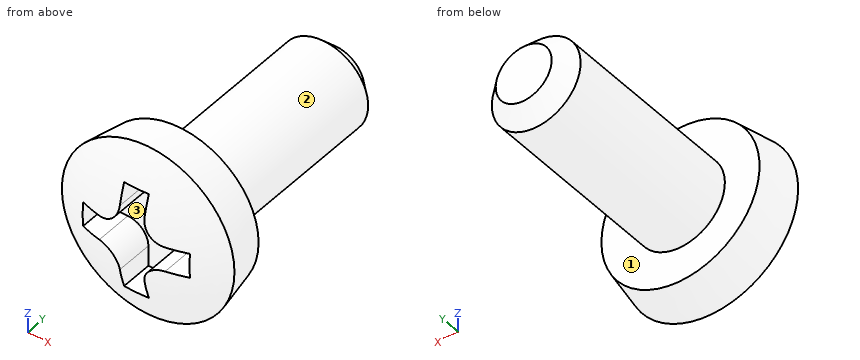
```python
from build123d import *

# Parameters (mm, degrees)
SKETCH1_R           = 2.667
BOSS_EXTRUDE1_DEPTH = 1.27
BOSS_EXTRUDE1_TAPER = 10
SKETCH3_R           = 1.3716
BOSS_EXTRUDE2_DEPTH = 6.35
CHAMFER1_SIZE       = 0.508
CUT_EXTRUDE5_DEPTH  = 3.048
FILLET1_R           = 0.635


with BuildPart() as part:
    # Sketch1 → Boss-Extrude1 (new body)
    with BuildSketch(Plane(origin=(0, 0, 0), x_dir=(1, 0, 0), z_dir=(0, 1, 0))):
        Circle(SKETCH1_R)
    extrude(amount=BOSS_EXTRUDE1_DEPTH, taper=BOSS_EXTRUDE1_TAPER)

    # Sketch2 → Revolve1 (revolve)
    with BuildSketch(Plane(origin=(0, 0, 0), x_dir=(0, 0, -1), z_dir=(1, 0, 0))):
        with BuildLine():
            Line((0, 0), (0, -0.762))
            ThreePointArc((0, -0.762), (-1.387624328, -0.57043515), (-2.667, 0))
            Line((-2.667, 0), (0, 0))
        make_face()
    revolve(axis=Axis((0, 0, 0), (0, -1, 0)))

    # Sketch3 → Boss-Extrude2 (add)
    with BuildSketch(Plane(origin=(0, 1.27, 0), x_dir=(1, 0, 0), z_dir=(0, 1, 0))):
        with Locations(Location((0, 0, 0), (0, 0, 270))):
            Circle(SKETCH3_R)
    extrude(amount=BOSS_EXTRUDE2_DEPTH)

    # Chamfer1
    chamfer1_edges = [part.edges().sort_by_distance(p)[0] for p in [
        (0, 7.62, -1.3716),
    ]]
    chamfer(chamfer1_edges, length=CHAMFER1_SIZE)

    # Sketch4 → Cut-Extrude5 (cut)
    with BuildSketch(Plane(origin=(0, -2.54, 0), x_dir=(1, 0, 0), z_dir=(0, 1, 0))):
        Polygon((-1.651, 0.381), (-1.651, -0.381), (-0.381, -0.381), (-0.381, -1.651), (0.381, -1.651), (0.381, -0.381), (1.651, -0.381), (1.651, 0.381), (0.381, 0.381), (0.381, 1.651), (-0.381, 1.651), (-0.381, 0.381), align=None)
    extrude(amount=CUT_EXTRUDE5_DEPTH, mode=Mode.SUBTRACT)

    # Fillet1
    fillet1_edges = [part.edges().sort_by_distance(p)[0] for p in [
        (0.381, -0.113446581, -0.381),
        (-0.381, -0.113446581, -0.381),
        (0.381, -0.113446581, 0.381),
        (-0.381, -0.113446581, 0.381),
    ]]
    fillet(fillet1_edges, radius=FILLET1_R)


solid = part.part
```
Read the model definition and answer for the solid it produces. Units are mm, in the model's axes. Face numbers are marked on the shaded views. Coordinates: 2 decimals unless noted, no trailing zeros. Loops run counter-clockwise (first coordinate to the right, second up) from the corner with the lowest first, then second, coordinate; pieces in that order, holes last. Notation, with made-up numbers: (17.5, 30.5) - (56.5, 30.5) arc R35 ccw to (56.5, 63.5) - close; hole circle Ø4 at (-11.5, 51.5). An arc over 180 degrees is marked (long way). Answer in a Markdown table with one row per item.
1. Straight lines are drawn through the part: line 1 (Z direction, x = -1.25, y = 0.25); line 2 (Y direction, x = -0.75, z = -0.05); line 3 (Y direction, x = 1.6, z = -0.7). For each, find the intervals that lie inside material, in ascending order.
Conclusion:
| item | result |
|---|---|
| line 1 | z = -2.31 to -0.38, 0.38 to 2.31 |
| line 2 | y = 0.51 to 7.62 |
| line 3 | y = -0.45 to 1.27 |
2. Find section A-A, the plane y = 1.75. Write down the section's boundary in (x, z).
Conclusion:
| item | result |
|---|---|
| outline | circle Ø2.74 at (0, 0) |
3. Determine the mould class of the marked faces 1, 2 and 3 for opening direction X: +X half, -X half, draft (parallel to the pull), parting line (faces both ways), or undercut.
Conclusion:
| item | result |
|---|---|
| face 1 | draft |
| face 2 | parting line |
| face 3 | undercut |
4. Given pin 1 (2 mm diameter, centred on x = 2, z = -1, fed in from -Y); pin 2 (1.5 mm diameter, centred on x = -1.5, y = 5, fed in from -Z); pin 3 (0.7 mm diameter, centred on y = 0, z = -1.5, fed in from +X), each flat-ended and moving along its own axis, determine where each tip first touches the part or whether it passes through.
Conclusion:
| item | result |
|---|---|
| pin 1 | stops at y = -0.61 |
| pin 2 | stops at z = -1.15 |
| pin 3 | stops at x = 2.41 |
